from build123d import *
from build123d.topology import SkipClean

# Parameters (mm, degrees)
SKETCH1_R               = 10
BOSS_EXTRUDE1_DEPTH     = 2
BOSS_EXTRUDE2_START     = -2
SKETCH2_R               = 2.55
BOSS_EXTRUDE2_DEPTH     = 2
CIRPATTERN1_COUNT       = 3
CUT_EXTRUDE1_DEPTH      = 27.9527328
SKETCH4_R               = 5.5
BOSS_EXTRUDE3_DEPTH     = 25
CUT_EXTRUDE2_START      = -7
SKETCH5_R               = 3
CUT_EXTRUDE2_DEPTH      = 7
CUT_EXTRUDE3_DEPTH      = 34.502982037
CUT_EXTRUDE3_DEPTH_BACK = 34.502982037
CUT_EXTRUDE4_START      = -7
SKETCH8_R               = 3.2
CUT_EXTRUDE4_DEPTH      = 7
FILLET2_R               = 5
CHAMFER1_START          = -2
CHAMFER1_2_DEPTH        = 2


with BuildPart() as part:
    # Sketch1 → Boss-Extrude1 (new body)
    with BuildSketch(Plane(origin=(0, 0, 0), x_dir=(1, 0, 0), z_dir=(0, 1, 0))):
        with Locations(Location((0, 0, 0), (0, 0, 270))):
            Circle(SKETCH1_R)
    extrude(amount=BOSS_EXTRUDE1_DEPTH)

    # Sketch2 → Boss-Extrude2 (add)
    with BuildSketch(Plane(origin=(0, 2, 0), x_dir=(1, 0, 0), z_dir=(0, 1, 0)).offset(BOSS_EXTRUDE2_START)):
        with BuildLine():
            Line((-4.75, 15.25), (-4.75, 8.799857953))
            ThreePointArc((-4.75, 8.799857953), (0, 10), (4.75, 8.799857953))
            Line((4.75, 8.799857953), (4.75, 15.25))
            ThreePointArc((4.75, 15.25), (0, 20), (-4.75, 15.25))
        make_face()
        with Locations(Location((0, 15.25, 0), (0, 0, 270))):
            Circle(SKETCH2_R, mode=Mode.SUBTRACT)
    boss_extrude2 = extrude(amount=BOSS_EXTRUDE2_DEPTH)

    # CirPattern1: Boss-Extrude2 ×3 about axis
    cirpattern1_axis = Axis((0, 0, 0), (0, 1, 0))
    for i in range(1, CIRPATTERN1_COUNT):
        add(boss_extrude2.rotate(cirpattern1_axis, i * 360 / CIRPATTERN1_COUNT))

    # Sketch3 → Cut-Extrude1 (cut, through all)
    with BuildSketch(Plane(origin=(0, 2, 0), x_dir=(1, 0, 0), z_dir=(0, 1, 0))):
        with BuildLine():
            Line((-2.653299832, 1.4), (2.653299832, 1.4))
            ThreePointArc((2.653299832, 1.4), (0, -3), (-2.653299832, 1.4))
        make_face()
    extrude(amount=-CUT_EXTRUDE1_DEPTH, mode=Mode.SUBTRACT)

    # Sketch4 → Boss-Extrude3 (add)
    with SkipClean():  # the faces are left unmerged after this step: merging them gives an invalid solid
        with BuildSketch(Plane.XZ):
            with Locations(Location((0, 0, 0), (0, 0, 90))):
                Circle(SKETCH4_R)
            with BuildLine():
                Line((2.653299832, -1.4), (-2.653299832, -1.4))
                ThreePointArc((-2.653299832, -1.4), (0, 3), (2.653299832, -1.4))
            make_face(mode=Mode.SUBTRACT)
        extrude(amount=BOSS_EXTRUDE3_DEPTH)

    # Sketch5 → Cut-Extrude2 (cut)
    with SkipClean():  # the faces are left unmerged after this step: merging them gives an invalid solid
        with BuildSketch(Plane.XZ.offset(25).offset(CUT_EXTRUDE2_START)):
            with Locations(Location((0, 0, 0), (0, 0, 332.181860715))):
                Circle(SKETCH5_R)
        extrude(amount=CUT_EXTRUDE2_DEPTH, mode=Mode.SUBTRACT)

    # Sketch7 → Cut-Extrude3 (cut, two sides: drawn at the far end of the back side and taken through both)
    with BuildSketch(Plane.XZ.offset(18).offset(-CUT_EXTRUDE3_DEPTH_BACK)):
        with BuildLine():
            Line((2.771281292, -1.6), (-2.771281292, -1.6))
            ThreePointArc((-2.771281292, -1.6), (0, 3.2), (2.771281292, -1.6))
        make_face()
        with BuildLine():
            Line((2.653299832, -1.4), (-2.653299832, -1.4))
            ThreePointArc((-2.653299832, -1.4), (0, 3), (2.653299832, -1.4))
        make_face(mode=Mode.SUBTRACT)
    extrude(amount=CUT_EXTRUDE3_DEPTH + CUT_EXTRUDE3_DEPTH_BACK, mode=Mode.SUBTRACT)

    # Sketch8 → Cut-Extrude4 (cut)
    with BuildSketch(Plane.XZ.offset(25).offset(CUT_EXTRUDE4_START)):
        with Locations(Location((0, 0, 0), (0, 0, 270))):
            Circle(SKETCH8_R)
    extrude(amount=CUT_EXTRUDE4_DEPTH, mode=Mode.SUBTRACT)

    # Fillet2
    fillet2_edges = [part.edges().sort_by_distance(p)[0] for p in [
        (9.995900537, 1, 0.286308309),
        (5.245900537, 1, 8.513549645),
        (-5.245900537, 1, 8.513549645),
        (-9.995900537, 1, 0.286308309),
        (-4.75, 1, -8.799857953),
        (4.75, 1, -8.799857953),
    ]]
    fillet(fillet2_edges, radius=FILLET2_R)

    # Chamfer1: read off the stored shape, not the designer's step
    # Chamfer1 outline → Chamfer1 (revolve)
    with BuildSketch(Plane.XY):
        Polygon((5.5, 0), (5.5, -5), (10.5, 0), align=None)
    revolve(axis=Axis((0, 0, 0), (0, 1, 0)))

    # Chamfer1 2 outline → Chamfer1 2 (cut)
    with BuildSketch(Plane(origin=(0, 0, 0), x_dir=(1, 0, 0), z_dir=(0, 1, 0)).offset(CHAMFER1_START)):
        with BuildLine():
            ThreePointArc((7.496834936, -9.813127226), (5.456150608, -9.164396031), (3.331223291, -9.428836163))
            ThreePointArc((3.331223291, -9.428836163), (0, -10), (-3.331223291, -9.428836163))
            ThreePointArc((-3.331223291, -9.428836163), (-5.456150608, -9.164396031), (-7.496834936, -9.813127226))
            Line((-7.496834936, -9.813127226), (-11.28460969, -12))
            Line((-11.28460969, -12), (11.28460969, -12))
            Line((11.28460969, -12), (7.496834936, -9.813127226))
        make_face()
        with BuildLine():
            ThreePointArc((9.831223291, 1.829494086), (10.582663547, -0.023370954), (12, -1.433664786))
            Line((12, -1.433664786), (12, 11))
            Line((12, 11), (4.765946576, 11))
            ThreePointArc((4.765946576, 11), (5.295673168, 9.12767596), (6.5, 7.599342077))
            ThreePointArc((6.5, 7.599342077), (8.660254038, 5), (9.831223291, 1.829494086))
        make_face()
        with BuildLine():
            Line((-12, 11), (-12, -1.433664786))
            ThreePointArc((-12, -1.433664786), (-10.582663547, -0.023370954), (-9.831223291, 1.829494086))
            ThreePointArc((-9.831223291, 1.829494086), (-8.660254038, 5), (-6.5, 7.599342077))
            ThreePointArc((-6.5, 7.599342077), (-5.295673168, 9.12767596), (-4.765946576, 11))
            Line((-4.765946576, 11), (-12, 11))
        make_face()
    extrude(amount=CHAMFER1_2_DEPTH, mode=Mode.SUBTRACT)


solid = part.part
The listing builds one solid part. Answer for the finished solid, in the listing's coordinates (mm). A direction names the side the tool comes from. Coordinates: 2 decimals unless noted, no trailing zeros. Write each loop counter-clockwise with the first axis right and the second up, starting at its lowest first coordinate (ties: lowest second). Pieces come first, ordered by that corner, then holes. Notation, with made-up numbers: (-34.75, 65) -> (-18.75, 65) arc R20 ccw to (-18.75, 101) -> close; hole circle Ø6 at (-30.5, 17.25). An arc over 180 degrees is marked (long way). One line per question, with ' | ' between items.
1. For a pull along Z with two mould halves and no side action, classify faces 6 (the cylindrical face through (17.267, 0.986, 10.09)), 7 (the flat face through (13.938, 0.986, 2.562)), 8 (the cylindrical face through (0.1, 1, -17.8)), 9 (the flat face through (-2, 0, -13)) as released by +Z, released by -Z, zero draft, split by the parting line, or undercut.
Verdict:
face 6: split by the parting line | face 7: released by -Z | face 8: undercut | face 9: zero draft
2. Section D-D (x = -1.5) is taken. State how many separate pieces and enclosed holes the cut face has, and give its area (3 significant figures).
Verdict:
separate pieces: 3 | enclosed holes: 0 | area: 213 mm^2
3. Section B-B (z = -17) is taken. Determine the outline of the cut face in (x, y).
Verdict:
outline: (-4.42, 0) -> (-1.85, 0) -> (-1.85, 2) -> (-4.42, 2) -> close; (1.85, 0) -> (4.42, 0) -> (4.42, 2) -> (1.85, 2) -> close
4. Given pin 1 Ø10 at (x, y) = (-1, -13.5) entering from +Z; pin 2 Ø3 at (x, z) = (1.5, -15.5) entering from -Y; pin 3 Ø0.5 at (x, z) = (1, -2) entering from -Y; pin 4 Ø6 at (x, z) = (9.5, -3.5) entering from +Y, each flat-ended and moving along its own axis, determine where each tip first touches the part or whether it passes through.
Verdict:
pin 1: stops at z = 5.5 | pin 2: stops at y = 0 | pin 3: stops at y = -18 | pin 4: stops at y = 2
5. Straight lines are drawn through the part: line 1 (X direction, y = 0.25, z = 8); line 2 (X direction, y = -11, z = 0); line 3 (Z direction, x = -2, y = -13.5). For each, find the intervals that lie inside material, in ascending order.
Verdict:
line 1: x = -17.94 to -15.73, -10.68 to 10.68, 15.73 to 17.94 | line 2: x = -5.5 to -3.2, 3.2 to 5.5 | line 3: z = -5.12 to -1.6, 2.5 to 5.12
6. Which of the six approach directions +Z, -Z, +X, -X, +Y, -Y give full straight-line access (tool end or side, diameter ignored) to faces 1 (the flat face through (-4.75, 1, -13)), 2 (the cylindrical face through (2.11, -14.86, 5.08)), 3 (the flat face through (4.75, 1, -13)), 4 (the flat face through (-9.19, 0.99, 10.79)), 5 (the flat face through (-10, 0, 7))?
Verdict:
face 1: -Z, -X, +Y, -Y | face 2: -Y | face 3: -Z, +X, +Y, -Y | face 4: +Z, +Y, -Y | face 5: +Z, -X, -Y
7. Section C-C (y = -3.25) is taken. Determine the outline of the cut face in (x, z).
Verdict:
outline: circle Ø14.5 at (0, 0); hole (-2.77, -1.6) -> (2.77, -1.6) arc R3.2 ccw (long way) to start
8. Section A-A (x = -14) is taken. Determine the outline of the cut face in (y, z), and give its area (3 significant figures).
Verdict:
outline: (0, 2.6) -> (2, 2.6) -> (2, 5.2) -> (0, 5.2) -> close; (0, 10.05) -> (2, 10.05) -> (2, 12.31) -> (0, 12.31) -> close | area: 9.73 mm^2
